Geometry check sheet. Reference: drawing and pictorial views, mm from the part's lowest x, y, z. A direction names the side the tool comes from. Round coordinates to 2 decimals unless told otherwise and drop trailing zeros. Write each loop counter-clockwise with the first axis right and the second up, starting at its lowest first coordinate (ties: lowest second). Pieces come first, ordered by that corner, then holes. Notation, with made-up numbers: (12, -12) -> (31, -12) arc R30 cw to (31, 25) -> close; hole circle Ø10 at (61.5, 83). An arc over 180 degrees is marked (long way). Answer as a JSON object with one key per item and string values. Group by question number.
(1) Set-up check for the marked faces 1, 2 and 3: record each of +Z, -Z, +X, -X, +Y, -Y from which the full face is reachable in a straight line by a thin tool's end or side.
(2) Sectioned sample at C-C on y = 2. Record the cut outline in (x, z) (1 decimal).
(3) Draft check along X on the marked faces 4, 5, 6 and 7. Enter one of: released by +X, released by -X, zero draft, split by the parting line, or undercut.
(4) Sectioned sample at B-B on z = 12.75. Record the cut outline in (x, y).
(5) Scan lines: L1, parallel to X at y = 1.25, z = 10.75; L2, parallel to Z at x = 22.5, y = 6.5; L3, parallel to X at y = 8, z = 16.5. Record each from-to range of solid material in increasing order. Write a range as from..to.
(6) Gauge pin test, flat ends, axial feed: pin 1 Ø1.6 at (x, y) = (5.5, 15) entering from +Z; pin 2 Ø4 at (y, z) = (10.5, 10.5) entering from +X. Record the tip position at first contact, or that the pin passes through.
(7) Sectioned sample at A-A on y = 11. Record the cut outline in (x, z) (1 decimal).
(8) Sectioned sample at D-D on z = 5.5. Record the cut outline in (x, y).
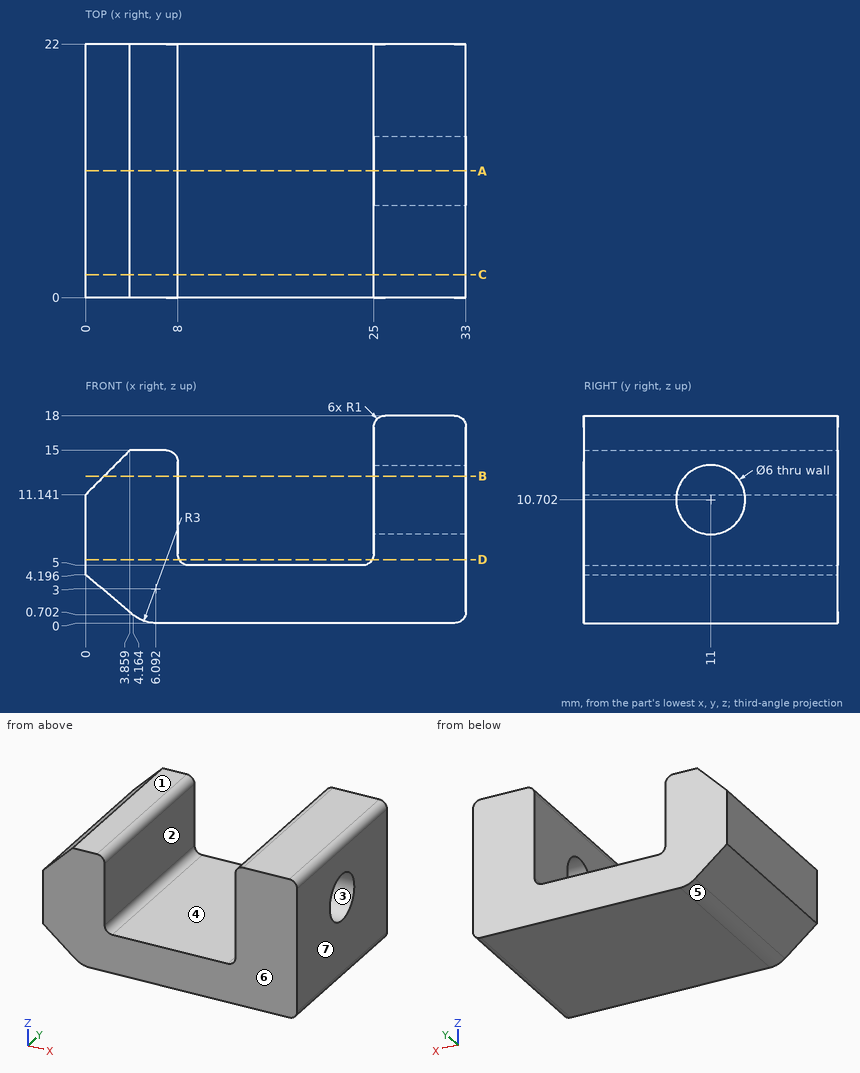
Computed values:
{
 "1": {"face 1": "+Z, -X, +Y, -Y", "face 2": "+Z, +Y, -Y", "face 3": "+X"},
 "2": {"outline": "(0, 4.2) -> (4.2, 0.7) arc R3 ccw to (6.1, 0) -> (32, 0) arc R1 ccw to (33, 1) -> (33, 17) arc R1 ccw to (32, 18) -> (26, 18) arc R1 ccw to (25, 17) -> (25, 6) arc R1 cw to (24, 5) -> (9, 5) arc R1 cw to (8, 6) -> (8, 14) arc R1 ccw to (7, 15) -> (3.9, 15) -> (0, 11.1) -> close"},
 "3": {"face 4": "undercut", "face 5": "released by -X", "face 6": "zero draft", "face 7": "released by +X"},
 "4": {"outline": "(1.61, 0) -> (8, 0) -> (8, 22) -> (1.61, 22) -> close; (25, 0) -> (33, 0) -> (33, 8.81) -> (25, 8.81) -> close; (25, 13.19) -> (33, 13.19) -> (33, 22) -> (25, 22) -> close"},
 "5": {"L1": "0..8, 25..33", "L2": "0..5", "L3": "25..33"},
 "6": {"pin 1": "z = 15", "pin 2": "x = 8"},
 "7": {"outline": "(0, 4.2) -> (4.2, 0.7) arc R3 ccw to (6.1, 0) -> (32, 0) arc R1 ccw to (33, 1) -> (33, 7.7) -> (25, 7.7) -> (25, 6) arc R1 cw to (24, 5) -> (9, 5) arc R1 cw to (8, 6) -> (8, 14) arc R1 ccw to (7, 15) -> (3.9, 15) -> (0, 11.1) -> close; (25, 13.7) -> (33, 13.7) -> (33, 17) arc R1 ccw to (32, 18) -> (26, 18) arc R1 ccw to (25, 17) -> close"},
 "8": {"outline": "(0, 0) -> (8.13, 0) -> (8.13, 22) -> (0, 22) -> close; (24.87, 0) -> (33, 0) -> (33, 22) -> (24.87, 22) -> close"}
}
